from build123d import *

# Parameters (mm, degrees)
SKETCH1_W           = 101.6
SKETCH1_H           = 101.6
BOSS_EXTRUDE1_DEPTH = 12.7
SKETCH7_W           = 63.5
SKETCH7_H           = 63.5
CUT_EXTRUDE2_DEPTH  = 6.35
SKETCH8_W           = 25.4
SKETCH8_H           = 6.35
CUT_EXTRUDE3_DEPTH  = 6.35
CIRPATTERN2_COUNT   = 4
BOSS_EXTRUDE3_START = -6.35
SKETCH9_W           = 31.75
SKETCH9_H           = 25.4
BOSS_EXTRUDE3_DEPTH = 6.35
CIRPATTERN3_COUNT   = 4


with BuildPart() as part:
    # Sketch1 → Boss-Extrude1 (new body)
    with BuildSketch(Plane(origin=(0, 0, 0), x_dir=(1, 0, 0), z_dir=(0, 1, 0))):
        with Locations((50.8, 50.8)):
            Rectangle(SKETCH1_W, SKETCH1_H)
    extrude(amount=BOSS_EXTRUDE1_DEPTH)

    # Sketch7 → Cut-Extrude2 (cut)
    with BuildSketch(Plane(origin=(0, 12.7, 0), x_dir=(1, 0, 0), z_dir=(0, 1, 0))):
        with Locations((50.8, 50.8)):
            Rectangle(SKETCH7_W, SKETCH7_H)
    extrude(amount=-CUT_EXTRUDE2_DEPTH, mode=Mode.SUBTRACT)

    # Sketch8 → Cut-Extrude3 (cut)
    with BuildSketch(Plane(origin=(0, 12.7, 0), x_dir=(1, 0, 0), z_dir=(0, 1, 0))):
        with Locations((50.8, 98.425)):
            Rectangle(SKETCH8_W, SKETCH8_H)
    cut_extrude3 = extrude(amount=-CUT_EXTRUDE3_DEPTH, mode=Mode.SUBTRACT)

    # CirPattern2: Cut-Extrude3 ×4 about axis
    cirpattern2_axis = Axis((50.8, 0, -50.8), (0, 1, 0))
    for i in range(1, CIRPATTERN2_COUNT):
        add(cut_extrude3.rotate(cirpattern2_axis, i * 360 / CIRPATTERN2_COUNT), mode=Mode.SUBTRACT)

    # Sketch9 → Boss-Extrude3 (add)
    with BuildSketch(Plane(origin=(0, 12.7, 0), x_dir=(1, 0, 0), z_dir=(0, 1, 0)).offset(BOSS_EXTRUDE3_START)):
        with Locations((50.8, 114.3)):
            Rectangle(SKETCH9_W, SKETCH9_H)
    boss_extrude3 = extrude(amount=-BOSS_EXTRUDE3_DEPTH)

    # CirPattern3: Boss-Extrude3 ×4 about axis
    cirpattern3_axis = Axis((50.8, 0, -50.8), (0, 1, 0))
    for i in range(1, CIRPATTERN3_COUNT):
        add(boss_extrude3.rotate(cirpattern3_axis, i * 360 / CIRPATTERN3_COUNT))


solid = part.part
Geometry check sheet. Reference: the model listing, model coordinates, mm. A direction names the side the tool comes from. Give positions to 0.01 mm unless a question says otherwise; leave off trailing zeros. Loops run counter-clockwise (first coordinate to the right, second up) from the corner with the lowest first, then second, coordinate; pieces in that order, holes last. Notation, with made-up numbers: M -13,15 L 43,15 A18 ccw 43,19 Z; hole C 0,69 d4. An arc over 180 degrees is marked long. Write each question's results on one line, items separated by ' | '.
1) Section check D-D, the plane z = -27. Record the boundary of the cut face in (x, y), plus the area to 3 significant figures.
Answers follow:
outline: M 0,0 L 101.6,0 L 101.6,12.7 L 82.55,12.7 L 82.55,6.35 L 19.05,6.35 L 19.05,12.7 L 0,12.7 Z | area: 887 mm2
2) Section check B-B, the plane x = 47. Record the boundary of the cut face in (y, z), plus the area to 3 significant figures.
Answers follow:
outline: M 0,-127 L 6.35,-127 L 6.35,-95.25 L 12.7,-95.25 L 12.7,-82.55 L 6.35,-82.55 L 6.35,-19.05 L 12.7,-19.05 L 12.7,-6.35 L 6.35,-6.35 L 6.35,25.4 L 0,25.4 Z | area: 1,130 mm2
3) Section check C-C, the plane z = -60.5. Record the boundary of the cut face in (x, y).
Answers follow:
outline: M -25.4,0 L 127,0 L 127,6.35 L 95.25,6.35 L 95.25,12.7 L 82.55,12.7 L 82.55,6.35 L 19.05,6.35 L 19.05,12.7 L 6.35,12.7 L 6.35,6.35 L -25.4,6.35 Z
4) Gauge pin test, flat ends, axial feed: pin 1 (5 mm diameter, centred on x = 14, y = 1.5, fed in from +Z); pin 2 (1.9 mm diameter, centred on x = 4.5, y = 9, fed in from -Z); pin 3 (5 mm diameter, centred on y = 3.5, z = 18, fed in from -X) (3 decimals). Record the tip position at first contact, or that the pin passes through.
Answers follow:
pin 1: z = 0 | pin 2: z = -101.6 | pin 3: x = 34.925
5) Section check A-A, the plane y = 10. Record the boundary of the cut face in (x, z), plus the area to 3 significant figures.
Answers follow:
outline: M 0,-101.6 L 38.1,-101.6 L 38.1,-95.25 L 63.5,-95.25 L 63.5,-101.6 L 101.6,-101.6 L 101.6,-63.5 L 95.25,-63.5 L 95.25,-38.1 L 101.6,-38.1 L 101.6,0 L 63.5,0 L 63.5,-6.35 L 38.1,-6.35 L 38.1,0 L 0,0 L 0,-38.1 L 6.35,-38.1 L 6.35,-63.5 L 0,-63.5 Z; hole M 19.05,-82.55 L 82.55,-82.55 L 82.55,-19.05 L 19.05,-19.05 Z | area: 5,650 mm2
6) Release check for a two-part mould opening along X. For faces 1 (the face through (66.675, 3, 13)), 2 (the face through (98, 10, -63.5)), 3 (the face through (50, 6.35, -51)) record: +X half, -X half, draft (parallel to the pull), parting line (faces both ways), or undercut.
Answers follow:
face 1: +X half | face 2: draft | face 3: undercut
7) Tool access check on faces 4 (the face through (82.55, 10, -50)), 5 (the face through (51, 10, -6.35)), 6 (the face through (98, 10, -38.1)), 7 (the face through (114, 3, -66.675)). Record the directions out of +Z, -Z, +X, -X, +Y, -Y that give a thin tool (end or side, any length) a straight path to the whole face; none if there is none.
Answers follow:
face 4: +Y | face 5: +Z, +Y | face 6: +X, +Y | face 7: -Z, +X, +Y, -Y
8) Thickness scan on line 1 (X direction, y = 8.75, z = -77); line 2 (Z direction, x = 77, y = 12); line 3 (X direction, y = 10.75, z = -1.5). Record the ranges inside material, lowest first.
Answers follow:
line 1: 0 to 19.05, 82.55 to 101.6 | line 2: -101.6 to -82.55, -19.05 to 0 | line 3: 0 to 38.1, 63.5 to 101.6
